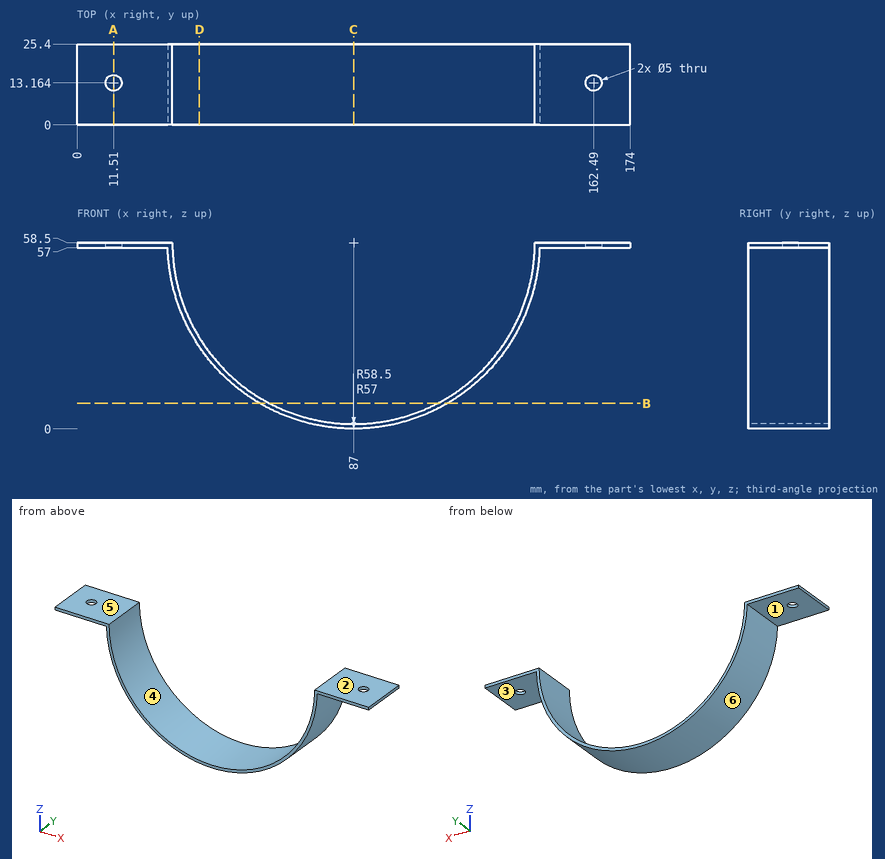
Study the drawing (mm; zero at the part's minimum x, y, z) and answer. A direction names the side the tool comes from. Coordinates: 2 decimals unless noted, no trailing zeros. Order: outer loops, then holes, each group sorted by start corner. A loop starts at its lowest first (then second) coordinate and runs counter-clockwise, first axis right, second up. Notation, with made-up numbers: (40, -17) -> (49, -17) arc R25 ccw to (49, 0) -> close; hole circle Ø6 at (47, 38). An arc over 180 degrees is marked (long way). Answer in a Markdown table with one row per item. Add a question column.
Item 1: Determine the mould class of the marked faces 4, 5 and 6 for opening direction X: +X half, -X half, draft (parallel to the pull), parting line (faces both ways), or undercut.
Item 2: Find section C-C (x = 87). Write down the section's boundary in (y, z).
Item 3: Which of the six approach directions +Z, -Z, +X, -X, +Y, -Y give full straight-line access (tool end or side, diameter ignored) to the marked faces 1, 2 and 3?
Item 4: Find section B-B (z = 8). Write down the section's boundary in (x, y).
Item 5: Each of these flat-tipped pins is pushed along its axis until it touches: P1, Ø4, axis at x = 39, y = 17.5, coming from the +Z side; P2, Ø7.5, axis at x = 163, y = 7, coming from the -Z side; P3, Ø2, axis at x = 90.5, y = 14.5, coming from the +Z side; P4, Ø12, axis at x = 152, z = 46, coming from the +Y side. Where does it stop, or does it pass through?
Item 6: Find the intervals of material crossed by L1, parallel to Z at x = 22.5, y = 17.5; L2, parallel to X at y = 24, z = 40 (1 decimal); L3, parallel to X at y = 5.5, z = 52.5, in increasing order. Write a range as from..to.
Item 7: Find section D-D (x = 38.5). Write down the section's boundary in (y, z).
Item 8: Find section A-A (x = 11.51). Write down the section's boundary in (y, z).
Result set:
| question | item | result |
|---|---|---|
| 1 | face 4 | undercut |
| 1 | face 5 | draft |
| 1 | face 6 | parting line |
| 2 | outline | (0, 0) -> (25.4, 0) -> (25.4, 1.5) -> (0, 1.5) -> close |
| 3 | face 1 | -Z, -X, +Y, -Y |
| 3 | face 2 | +Z, +X, -X, +Y, -Y |
| 3 | face 3 | -Z, +X, +Y, -Y |
| 4 | outline | (57.47, 0) -> (60.57, 0) -> (60.57, 25.4) -> (57.47, 25.4) -> close; (113.43, 0) -> (116.53, 0) -> (116.53, 25.4) -> (113.43, 25.4) -> close |
| 5 | P1 | stops at z = 31.13 |
| 5 | P2 | stops at z = 57 |
| 5 | P3 | stops at z = 1.68 |
| 5 | P4 | passes through |
| 6 | L1 | z = 57..58.5 |
| 6 | L2 | x = 31.5..33.1, 140.9..142.5 |
| 6 | L3 | x = 28.81..30.32, 143.68..145.19 |
| 7 | outline | (0, 25.79) -> (25.4, 25.79) -> (25.4, 28.55) -> (0, 28.55) -> close |
| 8 | outline | (0, 57) -> (10.66, 57) -> (10.66, 58.5) -> (0, 58.5) -> close; (15.66, 57) -> (25.4, 57) -> (25.4, 58.5) -> (15.66, 58.5) -> close |
